Could you check a few things on this drawing? It's one solid part, dimensions in mm from its lowest x, y, z. Coordinates: 2 decimals unless noted, no trailing zeros. Order: outer loops, then holes, each group sorted by start corner. A loop starts at its lowest first (then second) coordinate and runs counter-clockwise, first axis right, second up. Notation, with made-up numbers: M 8,61 L 54,61 A17 cw 54,84 Z; hole C 53,-3 d1. An arc over 180 degrees is marked long. Answer as CSV lines item,"result". Start each with the question number.
1. I need wall thicknesses on line 1 along Z through (x, y) = (6.5, 1.6) (1 decimal); line 2 along X through (y, z) = (0.2, 6.25) (1 decimal); line 3 along Z through (x, y) = (5.25, 1.5). Which ranges of each line are inside material? Lowest first, please. Write a range as from..to.
2. Will this pin go through, and if not, where does the flat tip stop? pin 1 (1 mm diameter, centred on y = 2, z = 9, fed in from +X).
3. If we section it at B-B (y = 0.95): List the corners of the cut face in (x, z) for me (1 decimal).
4. If we section it at A-A (y = 0.3): List the corners of the cut face in (x, z) for me.
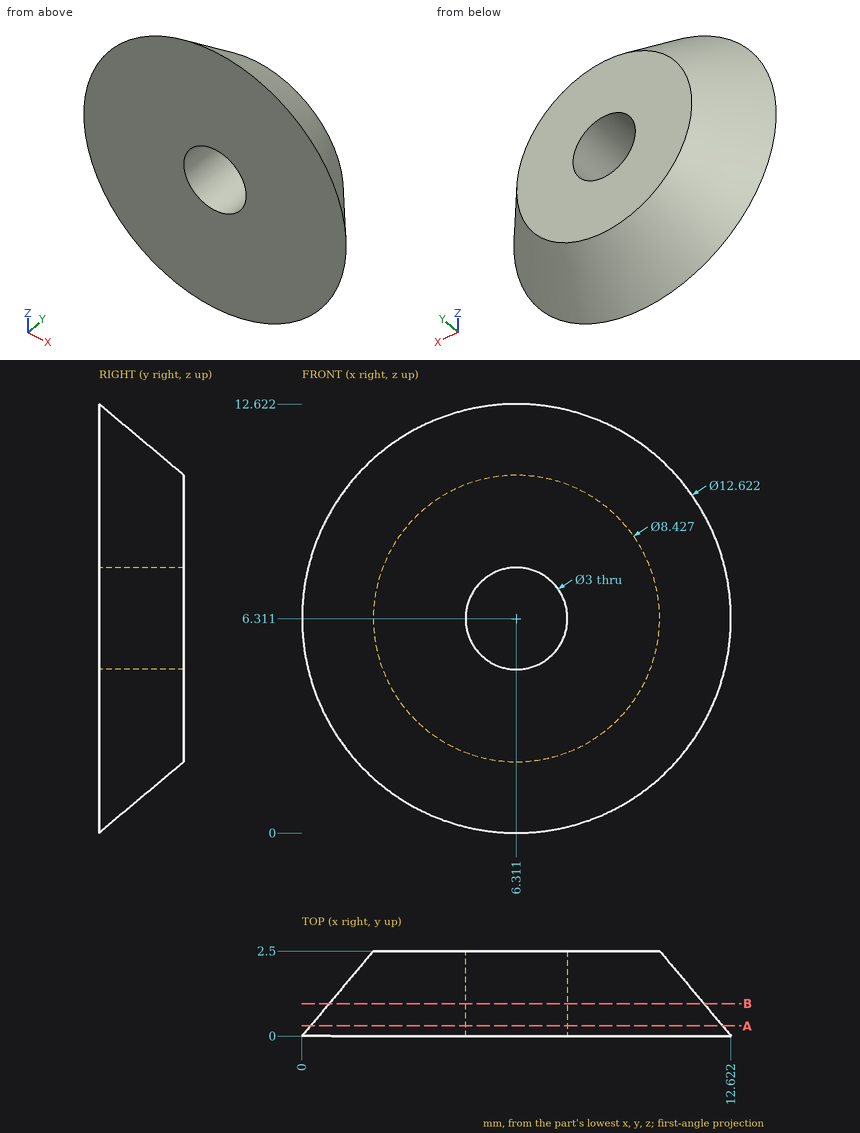
Solved:
1,line 1,"1.3..4.8, 7.8..11.3"
1,line 2,"0.2..4.8, 7.8..12.5"
1,line 3,"1.37..5.25, 7.37..11.25"
2,pin 1,"x = 10.67"
3,outline,"C 6.3,6.3 d11; hole C 6.3,6.3 d3"
4,outline,"C 6.31,6.31 d12.12; hole C 6.31,6.31 d3"
